Work out the finished part from the listing and answer in its coordinate system (mm). Round coordinates to 2 decimals unless told otherwise and drop trailing zeros. Order: outer loops, then holes, each group sorted by start corner. A loop starts at its lowest first (then second) coordinate and runs counter-clockwise, first axis right, second up. Notation, with made-up numbers: (17, 49.5) - (59, 49.5) arc R28 ccw to (59, 73.5) - close; hole circle Ø5 at (70.5, -34). An arc over 180 degrees is marked (long way). Use CSV: the item, a comma, the result in double quotes.
from build123d import *

# Parameters (mm, degrees)
SKETCH1_R           = 3.1
BOSS_EXTRUDE1_DEPTH = 3
CUT_EXTRUDE1_DEPTH  = 335.294780097
FILLET1_R           = 45
SKETCH3_R           = 12.6
CUT_EXTRUDE2_DEPTH  = 335.294780097
SKETCH4_R           = 2.5
CUT_EXTRUDE3_DEPTH  = 335.294780097
SKETCH5_W           = 15.2
SKETCH5_H           = 15.2
SKETCH5_W_2         = 0.2
CUT_EXTRUDE4_DEPTH  = 335.294780097
SKETCH10_R          = 2.6
SKETCH10_R_2        = 1.6
CUT_EXTRUDE8_DEPTH  = 335.294780097
FILLET2_R           = 10
FILLET3_R           = 2
SKETCH11_R          = 1.6
CUT_EXTRUDE9_DEPTH  = 335.294780097


with BuildPart() as part:
    # Sketch1 → Boss-Extrude1 (new body)
    # profile 1 of 2: a face of its own
    with BuildSketch(Plane(origin=(0, 0, 0), x_dir=(1, 0, 0), z_dir=(0, 1, 0))):
        with BuildLine():
            Line((0, -52), (260, -52))
            ThreePointArc((260, -52), (312, 0), (260, 52))
            Line((260, 52), (0, 52))
            ThreePointArc((0, 52), (-52, 0), (0, -52))
        make_face()
        with Locations(Location((0, 0, 0), (0, 0, 270))):
            Circle(SKETCH1_R, mode=Mode.SUBTRACT)
        with BuildLine():
            ThreePointArc((250, 3.1), (246.9, 0), (250, -3.1))
            Line((250, -3.1), (270, -3.1))
            ThreePointArc((270, -3.1), (273.1, 0), (270, 3.1))
            Line((270, 3.1), (250, 3.1))
        make_face(mode=Mode.SUBTRACT)
    # profile 2 of 2: a face of its own
    with BuildSketch(Plane(origin=(0, 0, 0), x_dir=(1, 0, 0), z_dir=(0, 1, 0))):
        with BuildLine():
            ThreePointArc((-52, 0), (-36.769552622, 36.769552622), (0, 52))
            Line((0, 52), (260, 52))
            ThreePointArc((260, 52), (296.769552622, 36.769552622), (312, 0))
            Line((312, 0), (312, 120))
            Line((312, 120), (-52, 120))
            Line((-52, 120), (-52, 0))
        make_face()
    extrude(amount=BOSS_EXTRUDE1_DEPTH)

    # Sketch2 → Cut-Extrude1 (cut, through all)
    with BuildSketch(Plane(origin=(0, 3, 0), x_dir=(1, 0, 0), z_dir=(0, 1, 0))):
        with BuildLine():
            Line((87.4, -37), (87.4, 98))
            ThreePointArc((87.4, 98), (90, 100.6), (92.6, 98))
            Line((92.6, 98), (92.6, -37))
            ThreePointArc((92.6, -37), (90, -39.6), (87.4, -37))
        make_face()
        with BuildLine():
            Line((172.6, -37), (172.6, 98))
            ThreePointArc((172.6, 98), (170, 100.6), (167.4, 98))
            Line((167.4, 98), (167.4, -37))
            ThreePointArc((167.4, -37), (170, -39.6), (172.6, -37))
        make_face()
    extrude(amount=-CUT_EXTRUDE1_DEPTH, mode=Mode.SUBTRACT)

    # Fillet1
    fillet1_edges = [part.edges().sort_by_distance(p)[0] for p in [
        (-52, 1.5, -120),
        (312, 1.5, -120),
    ]]
    fillet(fillet1_edges, radius=FILLET1_R)

    # Sketch3 → Cut-Extrude2 (cut, through all)
    with BuildSketch(Plane(origin=(0, 3, 0), x_dir=(1, 0, 0), z_dir=(0, 1, 0))):
        with Locations(Location((0, 0, 0), (0, 0, 270))):
            Circle(SKETCH3_R)
    extrude(amount=-CUT_EXTRUDE2_DEPTH, mode=Mode.SUBTRACT)

    # Sketch4 → Cut-Extrude3 (cut, through all)
    with BuildSketch(Plane(origin=(0, 3, 0), x_dir=(1, 0, 0), z_dir=(0, 1, 0))):
        with Locations(Location((-10.938925726, 19, 0), (0, 0, 270))):
            Circle(SKETCH4_R)
        with Locations(Location((45.07, 19, 0), (0, 0, 270))):
            Circle(SKETCH4_R)
        with Locations(Location((31.061074274, -19, 0), (0, 0, 270))):
            Circle(SKETCH4_R)
        with Locations(Location((-10.938925726, -19, 0), (0, 0, 270))):
            Circle(SKETCH4_R)
    extrude(amount=-CUT_EXTRUDE3_DEPTH, mode=Mode.SUBTRACT)

    # Sketch5 → Cut-Extrude4 (cut, through all)
    with BuildSketch(Plane(origin=(0, 3, 0), x_dir=(1, 0, 0), z_dir=(0, 1, 0))):
        with BuildLine():
            Line((-52, 108), (-37.594117082, 108))
            ThreePointArc((-37.594117082, 108), (-35.836098568, 109.546771476), (-34, 111))
            Line((-34, 111), (-52, 111))
            Line((-52, 111), (-52, 108))
        make_face()
        with BuildLine():
            Line((-37.594117082, 108), (-7.6, 108))
            Line((-7.6, 108), (7.6, 108))
            Line((7.6, 108), (7.8, 108))
            Line((7.8, 108), (7.8, 111))
            Line((7.8, 111), (-34, 111))
            ThreePointArc((-34, 111), (-35.836098568, 109.546771476), (-37.594117082, 108))
        make_face()
        with BuildLine():
            Line((-48.32989233, 92.8), (-7.6, 92.8))
            Line((-7.6, 92.8), (-7.6, 108))
            Line((-7.6, 108), (-37.594117082, 108))
            ThreePointArc((-37.594117082, 108), (-43.756302622, 100.961013415), (-48.32989233, 92.8))
        make_face()
        with BuildLine():
            Line((7.6, 92.8), (-7.6, 92.8))
            Line((-7.6, 92.8), (-48.32989233, 92.8))
            ThreePointArc((-48.32989233, 92.8), (-48.940072785, 91.310435149), (-49.496588098, 89.8))
            Line((-49.496588098, 89.8), (7.8, 89.8))
            Line((7.8, 89.8), (7.8, 92.8))
            Line((7.8, 92.8), (7.6, 92.8))
        make_face()
        with BuildLine():
            Line((-52, 92.8), (-48.32989233, 92.8))
            ThreePointArc((-48.32989233, 92.8), (-43.756302622, 100.961013415), (-37.594117082, 108))
            Line((-37.594117082, 108), (-52, 108))
            Line((-52, 108), (-52, 92.8))
        make_face()
        with BuildLine():
            ThreePointArc((-49.496588098, 89.8), (-48.940072785, 91.310435149), (-48.32989233, 92.8))
            Line((-48.32989233, 92.8), (-52, 92.8))
            Line((-52, 92.8), (-52, 89.8))
            Line((-52, 89.8), (-49.496588098, 89.8))
        make_face()
        with Locations((0, 100.4)):
            Rectangle(SKETCH5_W, SKETCH5_H)
        with Locations((7.7, 100.4)):
            Rectangle(SKETCH5_W_2, SKETCH5_H)
        with BuildLine():
            Line((252.2, 108), (252.4, 108))
            Line((252.4, 108), (267.6, 108))
            Line((267.6, 108), (297.594117082, 108))
            ThreePointArc((297.594117082, 108), (295.836098568, 109.546771476), (294, 111))
            Line((294, 111), (252.2, 111))
            Line((252.2, 111), (252.2, 108))
        make_face()
        with Locations((260, 100.4)):
            Rectangle(SKETCH5_W, SKETCH5_H)
        with Locations((252.3, 100.4)):
            Rectangle(SKETCH5_W_2, SKETCH5_H)
        with BuildLine():
            Line((267.6, 92.8), (252.4, 92.8))
            Line((252.4, 92.8), (252.2, 92.8))
            Line((252.2, 92.8), (252.2, 89.8))
            Line((252.2, 89.8), (309.496588098, 89.8))
            ThreePointArc((309.496588098, 89.8), (308.940072785, 91.310435149), (308.32989233, 92.8))
            Line((308.32989233, 92.8), (267.6, 92.8))
        make_face()
        with BuildLine():
            Line((297.594117082, 108), (267.6, 108))
            Line((267.6, 108), (267.6, 92.8))
            Line((267.6, 92.8), (308.32989233, 92.8))
            ThreePointArc((308.32989233, 92.8), (303.756302622, 100.961013415), (297.594117082, 108))
        make_face()
        with BuildLine():
            ThreePointArc((294, 111), (295.836098568, 109.546771476), (297.594117082, 108))
            Line((297.594117082, 108), (312, 108))
            Line((312, 108), (312, 111))
            Line((312, 111), (294, 111))
        make_face()
        with BuildLine():
            Line((312, 108), (297.594117082, 108))
            ThreePointArc((297.594117082, 108), (303.756302622, 100.961013415), (308.32989233, 92.8))
            Line((308.32989233, 92.8), (312, 92.8))
            Line((312, 92.8), (312, 108))
        make_face()
        with BuildLine():
            Line((312, 92.8), (308.32989233, 92.8))
            ThreePointArc((308.32989233, 92.8), (308.940072785, 91.310435149), (309.496588098, 89.8))
            Line((309.496588098, 89.8), (312, 89.8))
            Line((312, 89.8), (312, 92.8))
        make_face()
    extrude(amount=-CUT_EXTRUDE4_DEPTH, mode=Mode.SUBTRACT)

    # Sketch10 → Cut-Extrude8 (cut, through all)
    with BuildSketch(Plane(origin=(0, 3, 0), x_dir=(1, 0, 0), z_dir=(0, 1, 0))):
        with Locations(Location((17.4, 100.4, 0), (0, 0, 270))):
            Circle(SKETCH10_R)
        with Locations(Location((27.4, 100.4, 0), (0, 0, 270))):
            Circle(SKETCH10_R)
        with Locations(Location((242.4, 100.4, 0), (0, 0, 270))):
            Circle(SKETCH10_R)
        with Locations(Location((232.4, 100.4, 0), (0, 0, 270))):
            Circle(SKETCH10_R)
        with Locations(Location((207.4, 100.4, 0), (0, 0, 270))):
            Circle(SKETCH10_R_2)
        with Locations(Location((177.4, 100.4, 0), (0, 0, 270))):
            Circle(SKETCH10_R_2)
        with Locations(Location((147.4, 100.4, 0), (0, 0, 270))):
            Circle(SKETCH10_R_2)
        with Locations(Location((112.4, 100.4, 0), (0, 0, 270))):
            Circle(SKETCH10_R_2)
        with Locations(Location((52.4, 100.4, 0), (0, 0, 270))):
            Circle(SKETCH10_R_2)
        with Locations(Location((82.4, 100.4, 0), (0, 0, 270))):
            Circle(SKETCH10_R_2)
    extrude(amount=-CUT_EXTRUDE8_DEPTH, mode=Mode.SUBTRACT)

    # Fillet2
    fillet2_edges = [part.edges().sort_by_distance(p)[0] for p in [
        (-49.496588098, 1.5, -89.8),
        (309.496588098, 1.5, -89.8),
    ]]
    fillet(fillet2_edges, radius=FILLET2_R)

    # Fillet3
    fillet3_edges = [part.edges().sort_by_distance(p)[0] for p in [
        (-34, 1.5, -111),
        (294, 1.5, -111),
    ]]
    fillet(fillet3_edges, radius=FILLET3_R)

    # Sketch11 → Cut-Extrude9 (cut, through all)
    with BuildSketch(Plane.XZ):
        with Locations(Location((231.4, -12.4, 0), (0, 0, 270))):
            Circle(SKETCH11_R)
        with Locations(Location((198.4, -12.4, 0), (0, 0, 270))):
            Circle(SKETCH11_R)
    extrude(amount=-CUT_EXTRUDE9_DEPTH, mode=Mode.SUBTRACT)


solid = part.part
(1) Find the intervals of material crossed by L1, parallel to Z at x = 254, y = 2.7; L2, parallel to X at y = 2.1, z = 0; L3, parallel to X at y = 1.2, z = -27, in increasing order. Write a range as from..to.
Findings below:
L1,"z = -120..-111, -89.8..-3.1, 3.1..52"
L2,"x = -52..-12.6, 12.6..87.4, 92.6..167.4, 172.6..246.9, 273.1..312"
L3,"x = -52..87.4, 92.6..167.4, 172.6..312"
(2) The mould has two halves that part along Z. Classify faces 1 (the cylindrical face through (-7.667, 1.521, -9.999)), 2 (the cylindrical face through (308.313, 1.521, -87.274)), 3 (the flat face through (127, 3, -35)), 4 (the cylindrical face through (-37.172, 1.479, 36.363)): released by +Z, released by -Z, zero draft, split by the parting line, or undercut.
Findings below:
face 1,"undercut"
face 2,"released by -Z"
face 3,"zero draft"
face 4,"released by +Z"
(3) This flat-tipped pin is pushed along its axis until it touches: pin 1 (0.9 mm diameter, centred on y = 1, z = -100, fed in from -X). Where does it stop, or does it pass through?
Findings below:
pin 1,"stops at x = 7.8"
(4) Find section A-A (z = -38). Determine the outline of the cut face in (x, y), and give its area (3 significant figures).
Findings below:
outline,"(-52, 0) - (87.4, 0) - (87.4, 3) - (-52, 3) - close; (92.6, 0) - (167.4, 0) - (167.4, 3) - (92.6, 3) - close; (172.6, 0) - (312, 0) - (312, 3) - (172.6, 3) - close"
area,"1,060 mm²"
(5) Find section C-C (y = 0.9). State how many separate pieces and enclosed holes the cut face has, and give its area (3 significant figures).
Findings below:
separate pieces,"1"
enclosed holes,"20"
area,"56,000 mm²"
(6) Find section B-B (x = 280). Determine the outline of the cut face in (y, z).
Findings below:
outline,"(0, -118.08) - (3, -118.08) - (3, -111) - (0, -111) - close; (0, -89.8) - (3, -89.8) - (3, 48) - (0, 48) - close"
